```python
from build123d import *

# Parameters (mm, degrees)
SKETCH_R     = 1.5
PAD_DEPTH    = 452
PAD001_DEPTH = 5.08
SKETCH002_W  = 42
SKETCH002_H  = 60
PAD002_DEPTH = 5


with BuildPart() as part:
    # Sketch → Pad (new body, symmetric)
    with BuildSketch(Plane.YZ):
        Polygon((-10, 30), (-3, 30), (-3, 28.5), (-4.5, 28.5), (-4.5, 27), (-1.5, 24), (1.5, 24), (4.5, 27), (4.5, 28.5), (3, 28.5), (3, 30), (10, 30), (10, 25), (8.5, 25), (8.5, 26.5), (7, 26.5), (4, 23.5), (4, 20.5), (7, 17.5), (8.5, 17.5), (8.5, 19), (10, 19), (10, 11), (8.5, 11), (8.5, 12.5), (7, 12.5), (4, 9.5), (4, 6.5), (7, 3.5), (8.5, 3.5), (8.5, 5), (10, 5), (10, 0), (3, 0), (3, 1.5), (4.5, 1.5), (4.5, 3), (1.5, 6), (-1.5, 6), (-4.5, 3), (-4.5, 1.5), (-3, 1.5), (-3, 0), (-10, 0), (-10, 5), (-8.5, 5), (-8.5, 3.5), (-7, 3.5), (-4, 6.5), (-4, 9.5), (-7, 12.5), (-8.5, 12.5), (-8.5, 11), (-10, 11), (-10, 19), (-8.5, 19), (-8.5, 17.5), (-7, 17.5), (-4, 20.5), (-4, 23.5), (-7, 26.5), (-8.5, 26.5), (-8.5, 25), (-10, 25), align=None)
        with Locations((0, 8)):
            Circle(SKETCH_R, mode=Mode.SUBTRACT)
        with Locations((0, 22)):
            Circle(SKETCH_R, mode=Mode.SUBTRACT)
        Polygon((-7, 15), (-2.716354, 19.283646), (2.716354, 19.283646), (7, 15), (2.716354, 10.716354), (-2.716354, 10.716354), align=None, mode=Mode.SUBTRACT)
    extrude(amount=PAD_DEPTH, both=True)

    # Sketch001 → Pad001 (join)
    with BuildSketch(Plane.YZ.offset(452)):
        Polygon((-33, 68.5), (-33, 21.5), (-58, 21.5), (-58, -21.5), (-37, -21.5), (-37, -42.5), (-13.928203, -42.5), (-7, -38.5), (14, -38.5), (20.928203, -42.5), (37, -42.5), (37, -21.5), (58, -21.5), (58, 68.5), align=None)
    pad001 = extrude(amount=PAD001_DEPTH)

    # Mirrored: Pad001 across YZ
    add(pad001.mirror(Plane.YZ))

    # Sketch002 → Pad002 (join)
    with BuildSketch(Plane.XZ.offset(-10)):
        with Locations((404, -0.3)):
            Rectangle(SKETCH002_W, SKETCH002_H)
    extrude(amount=-PAD002_DEPTH)


solid = part.part
```
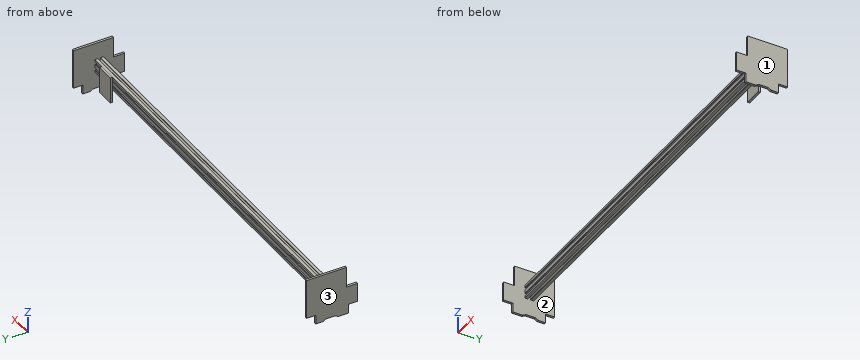
Work out the finished part from the listing and answer in its coordinate system (mm). Face numbers are marked on the shaded views. Coordinates: 2 decimals unless noted, no trailing zeros. Loops run counter-clockwise (first coordinate to the right, second up) from the corner with the lowest first, then second, coordinate; pieces in that order, holes last.
1) Consider probe 1 along Z at (x, y) = (166, 0); probe 2 along Y at (x, z) = (280, 3); probe 3 along X at (y, z) = (28.5, 33). Determine where each line is inside the solid, lowest interval first.
Results:
probe 1: z = 6 to 6.5, 9.5 to 10.72, 19.28 to 20.5, 23.5 to 24
probe 2: y = -10 to -4.5, 4.5 to 10
probe 3: x = -457.08 to -452, 452 to 457.08
2) For a pull along X with two mould halves and no side action, classify the marked faces 1, 2 and 3 as +X half, -X half, draft (parallel to the pull), parting line (faces both ways), or undercut.
Results:
face 1: +X half
face 2: undercut
face 3: -X half
3) Section C-C (x = 280) is taken. Give the number of separate pieces and of enclosed holes in the cut face, plus the area to 3 significant figures.
Results:
separate pieces: 1
enclosed holes: 3
area: 260 mm2
4) Section A-A (y = -23) is taken. Give the vertices of the cut face in (x, z).
Results:
outline: (-457.08, -42.5) - (-452, -42.5) - (-452, 68.5) - (-457.08, 68.5) - close; (452, -42.5) - (457.08, -42.5) - (457.08, 68.5) - (452, 68.5) - close
5) Flat-ended cylindrical pins translate along their axes: pin 1 (0.8 mm diameter, centred on x = -11, z = 29, fed in from -Y); pin 2 (1.5 mm diameter, centred on x = 29, z = -2, fed in from -Y); pin 3 (5.5 mm diameter, centred on x = 400, y = 13.5, fed in from -Z); pin 4 (5.5 mm diameter, centred on x = -453.5, y = -48, fed in from +Z). Find the tip coordinate at first contact, or state that the pin passes through.
Results:
pin 1: stops at y = -10
pin 2: passes through
pin 3: stops at z = -30.3
pin 4: stops at z = 21.5
6) Section B-B (z = 39) is taken. Give the vertices of the cut face in (x, y).
Results:
outline: (-457.08, -33) - (-452, -33) - (-452, 58) - (-457.08, 58) - close; (452, -33) - (457.08, -33) - (457.08, 58) - (452, 58) - close
